Input: dimensioned drawing with shaded views. Units: mm. Origin: part minimum x, y, z. A direction names the side the tool comes from. Coordinates: 2 decimals unless noted, no trailing zeros. Order: outer loops, then holes, each group sorted by start corner. A loop starts at its lowest first (then second) coordinate and runs counter-clockwise, first axis right, second up. Notation, with made-up numbers: (47, 86.5) -> (101, 86.5) arc R14 cw to (101, 90.5) -> close; hole circle Ø2 at (-13, 43.25). An arc over 180 degrees is marked (long way). Answer in a Markdown table with one row per item. Add a question column.
1) Section query A-A on y = 56.5. Return the cut outline in (x, z).
2) Set-up query: the marked faces 1, 2 and 3. Return all of +Z, -Z, +X, -X, +Y, -Y with unobstructed straight access to the full face (end or side cutting, diameter ignored); none if empty.
3) Pull-direction query (Y, two-part tool) for the marked faces 4, 5 and 6; classes: +Y half, -Y half, draft (parallel to the pull), parting line (faces both ways), or undercut.
4) Section query C-C on x = 79.5. Return the cut outline in (y, z).
5) Ray query, line 1 (X direction, y = 7.5, z = 5.45); line 2 (Y direction, x = 29.5, z = 6.5); line 3 (Z direction, x = 8.5, y = 57). Return the intervals inside material, ascending. Write a range as from..to.
6) Section query B-B on z = 7. Return the cut outline in (x, y), then the cut area to 3 significant figures.
7) Section query D-D on x = 48.5. Return the cut outline in (y, z), then the cut area to 3 significant figures.
8) Contact query for flat-ended pins moving along their axis: P1, Ø4, axis at x = 96, y = 5, coming from the -Z side; P2, Ø3.5, axis at x = 59, y = 39.5, coming from the -Z side; P3, Ø2.5, axis at x = 21.5, y = 7.5, coming from the +Z side; P4, Ø0.5, axis at x = 47.5, z = 0.5, coming from the -Y side. Output: stop coordinate, or through.
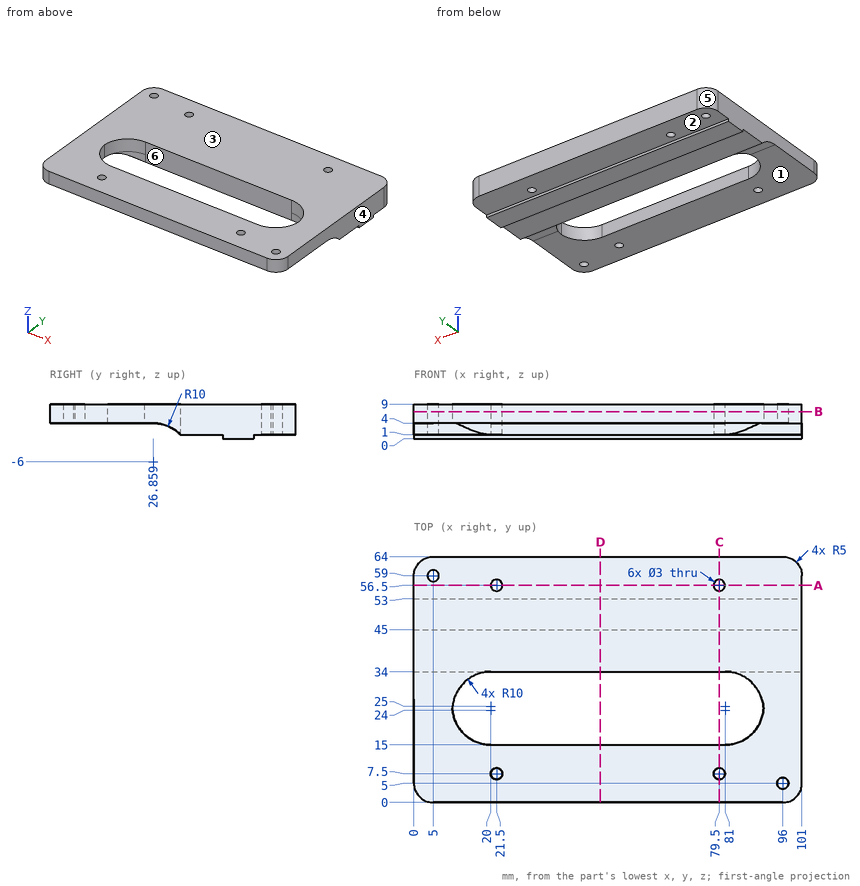
Result:
| question | item | result |
|---|---|---|
| 1 | outline | (0, 1) -> (20, 1) -> (20, 9) -> (0, 9) -> close; (23, 1) -> (78, 1) -> (78, 9) -> (23, 9) -> close; (81, 1) -> (101, 1) -> (101, 9) -> (81, 9) -> close |
| 2 | face 1 | -Z, +X, -X, -Y |
| 2 | face 2 | -Z, +X, -X, +Y |
| 2 | face 3 | +Z, +X, -X, +Y, -Y |
| 3 | face 4 | draft |
| 3 | face 5 | +Y half |
| 3 | face 6 | undercut |
| 4 | outline | (0, 4) -> (6, 4) -> (6, 9) -> (0, 9) -> close; (9, 4) -> (15, 4) -> (15, 9) -> (9, 9) -> close; (34, 1) -> (45, 1) -> (45, 0) -> (53, 0) -> (53, 1) -> (55, 1) -> (55, 9) -> (34, 9) -> close; (58, 1) -> (64, 1) -> (64, 9) -> (58, 9) -> close |
| 5 | line 1 | 0..20, 23..78, 81..101 |
| 5 | line 2 | 0..15, 34..64 |
| 5 | line 3 | 1..9 |
| 6 | outline | (0, 5) arc R5 ccw to (5, 0) -> (96, 0) arc R5 ccw to (101, 5) -> (101, 59) arc R5 ccw to (96, 64) -> (5, 64) arc R5 ccw to (0, 59) -> close; hole circle Ø3 at (5, 59); hole (10.01, 24.5) arc R10 ccw to (20, 15) -> (81, 15) arc R10 ccw to (90.99, 24.5) arc R10 ccw to (81, 34) -> (20, 34) arc R10 ccw to start; hole circle Ø3 at (21.5, 7.5); hole circle Ø3 at (21.5, 56.5); hole circle Ø3 at (79.5, 7.5); hole circle Ø3 at (79.5, 56.5); hole circle Ø3 at (96, 5) |
| 6 | area | 4,950 mm2 |
| 7 | outline | (0, 4) -> (15, 4) -> (15, 9) -> (0, 9) -> close; (34, 1) -> (45, 1) -> (45, 0) -> (53, 0) -> (53, 1) -> (64, 1) -> (64, 9) -> (34, 9) -> close |
| 7 | area | 323 mm2 |
| 8 | P1 | z = 4 |
| 8 | P2 | z = 1 |
| 8 | P3 | through |
| 8 | P4 | y = 45 |
